Model file for the job. Use its own axes, mm. A direction names the side the tool comes from. Round coordinates to 2 decimals unless told otherwise and drop trailing zeros. Loops run counter-clockwise (first coordinate to the right, second up) from the corner with the lowest first, then second, coordinate; pieces in that order, holes last. Notation, with made-up numbers: (6.25, -11.75) - (37.25, -11.75) arc R20 cw to (37.25, 15.25) - close; hole circle Ø8 at (68, 87.25). An arc over 180 degrees is marked (long way). Answer as a JSON object with one key per item and string values.
from build123d import *

# Parameters (mm, degrees)
F0_R     = 3
F0_R_2   = 1.9
F0_R_3   = 1.2
F1_DEPTH = 2
F2_R     = 3
F2_R_2   = 1.9
F3_DEPTH = 1
F4_R     = 3
F5_DEPTH = 0.5
F6_R     = 3
F7_DEPTH = 3
F8_DEPTH = 5


with BuildPart() as f1:
    # F0 (on Top) → F1 (new body)
    with BuildSketch(Plane.XY):
        with Locations((-10.4432452041, 0)):
            Circle(F0_R)
        with Locations((-10.4432452041, 0)):
            Circle(F0_R_2, mode=Mode.SUBTRACT)
        with Locations((-10.4432452041, 0)):
            Circle(F0_R_2)
        with Locations((-10.4432452041, 0)):
            Circle(F0_R_3, mode=Mode.SUBTRACT)
        with Locations((-10.4432452041, 0)):
            Circle(F0_R_3)
    extrude(amount=F1_DEPTH)

    # F2 (on face) → F3 (join)
    with BuildSketch(Plane.XY.offset(2)):
        with Locations((-10.4432452041, 0)):
            Circle(F2_R)
        with Locations((-10.4432452041, 0)):
            Circle(F2_R_2, mode=Mode.SUBTRACT)
    extrude(amount=F3_DEPTH)

    # F4 (on face) → F5 (join)
    with BuildSketch(Plane.XY.offset(3)):
        with Locations((-10.4432452041, 0)):
            Circle(F4_R)
        with BuildLine():
            ThreePointArc((-12.2866257343, 0.4603783455), (-10.4432452041, 1.9), (-8.5998646739, 0.4603783455))
            Line((-8.5998646739, 0.4603783455), (-7.8815174605, 0.4603783455))
            Line((-7.8815174605, 0.4603783455), (-7.8815174605, -0.4603783455))
            Line((-7.8815174605, -0.4603783455), (-8.5998646739, -0.4603783455))
            ThreePointArc((-8.5998646739, -0.4603783455), (-10.4432452041, -1.9), (-12.2866257343, -0.4603783455))
            Line((-12.2866257343, -0.4603783455), (-12.7640617396, -0.4603783455))
            Line((-12.7640617396, -0.4603783455), (-12.7640617396, 0.4603783455))
            Line((-12.7640617396, 0.4603783455), (-12.2866257343, 0.4603783455))
        make_face(mode=Mode.SUBTRACT)
        with BuildLine():
            ThreePointArc((-12.2866257343, -0.4603783455), (-12.3432452041, 0), (-12.2866257343, 0.4603783455))
            Line((-12.2866257343, 0.4603783455), (-12.7640617396, 0.4603783455))
            Line((-12.7640617396, 0.4603783455), (-12.7640617396, -0.4603783455))
            Line((-12.7640617396, -0.4603783455), (-12.2866257343, -0.4603783455))
        make_face()
        with BuildLine():
            ThreePointArc((-11.5514201808, -0.4603783455), (-11.6432452041, 0), (-11.5514201808, 0.4603783455))
            Line((-11.5514201808, 0.4603783455), (-12.2866257343, 0.4603783455))
            ThreePointArc((-12.2866257343, 0.4603783455), (-12.3432452041, 0), (-12.2866257343, -0.4603783455))
            Line((-12.2866257343, -0.4603783455), (-11.5514201808, -0.4603783455))
        make_face()
        with BuildLine():
            ThreePointArc((-9.3350702274, -0.4603783455), (-9.2664253428, -0.234723271), (-9.2432452041, 0))
            ThreePointArc((-9.2432452041, 0), (-9.2664253428, 0.234723271), (-9.3350702274, 0.4603783455))
            Line((-9.3350702274, 0.4603783455), (-11.5514201808, 0.4603783455))
            ThreePointArc((-11.5514201808, 0.4603783455), (-11.6432452041, 0), (-11.5514201808, -0.4603783455))
            Line((-11.5514201808, -0.4603783455), (-9.3350702274, -0.4603783455))
        make_face()
        with BuildLine():
            Line((-11.5514201808, 0.4603783455), (-9.3350702274, 0.4603783455))
            ThreePointArc((-9.3350702274, 0.4603783455), (-10.4432452041, 1.2), (-11.5514201808, 0.4603783455))
        make_face()
        with BuildLine():
            ThreePointArc((-11.5514201808, -0.4603783455), (-10.4432452041, -1.2), (-9.3350702274, -0.4603783455))
            Line((-9.3350702274, -0.4603783455), (-11.5514201808, -0.4603783455))
        make_face()
        with BuildLine():
            ThreePointArc((-9.3350702274, 0.4603783455), (-9.2664253428, 0.234723271), (-9.2432452041, 0))
            ThreePointArc((-9.2432452041, 0), (-9.2664253428, -0.234723271), (-9.3350702274, -0.4603783455))
            Line((-9.3350702274, -0.4603783455), (-8.5998646739, -0.4603783455))
            ThreePointArc((-8.5998646739, -0.4603783455), (-8.5574531944, -0.2319234708), (-8.5432452041, 0))
            ThreePointArc((-8.5432452041, 0), (-8.5574531944, 0.2319234708), (-8.5998646739, 0.4603783455))
            Line((-8.5998646739, 0.4603783455), (-9.3350702274, 0.4603783455))
        make_face()
        with BuildLine():
            Line((-7.8815174605, 0.4603783455), (-8.5998646739, 0.4603783455))
            ThreePointArc((-8.5998646739, 0.4603783455), (-8.5574531944, 0.2319234708), (-8.5432452041, 0))
            ThreePointArc((-8.5432452041, 0), (-8.5574531944, -0.2319234708), (-8.5998646739, -0.4603783455))
            Line((-8.5998646739, -0.4603783455), (-7.8815174605, -0.4603783455))
            Line((-7.8815174605, -0.4603783455), (-7.8815174605, 0.4603783455))
        make_face()
    extrude(amount=F5_DEPTH)

    # F6 (on face) → F7 (join)
    with BuildSketch(Plane.XY.offset(3.5)):
        with Locations((-10.4432452041, 0)):
            Circle(F6_R)
        with BuildLine():
            ThreePointArc((-12.2866257343, 0.4603783455), (-10.4432452041, 1.9), (-8.5998646739, 0.4603783455))
            ThreePointArc((-8.5998646739, 0.4603783455), (-8.5574531944, 0.2319234708), (-8.5432452041, 0))
            ThreePointArc((-8.5432452041, 0), (-8.5574531944, -0.2319234708), (-8.5998646739, -0.4603783455))
            ThreePointArc((-8.5998646739, -0.4603783455), (-10.4432452041, -1.9), (-12.2866257343, -0.4603783455))
            ThreePointArc((-12.2866257343, -0.4603783455), (-12.3432452041, 0), (-12.2866257343, 0.4603783455))
        make_face(mode=Mode.SUBTRACT)
        with BuildLine():
            ThreePointArc((-9.3350702274, -0.4603783455), (-9.2664253428, -0.234723271), (-9.2432452041, 0))
            ThreePointArc((-9.2432452041, 0), (-9.2664253428, 0.234723271), (-9.3350702274, 0.4603783455))
            ThreePointArc((-9.3350702274, 0.4603783455), (-10.4432452041, 1.2), (-11.5514201808, 0.4603783455))
            ThreePointArc((-11.5514201808, 0.4603783455), (-11.6432452041, 0), (-11.5514201808, -0.4603783455))
            ThreePointArc((-11.5514201808, -0.4603783455), (-10.4432452041, -1.2), (-9.3350702274, -0.4603783455))
        make_face()
    extrude(amount=F7_DEPTH)

    # F8 (add): a face of the model
    f8_faces = [f1.faces().sort_by_distance(p)[0] for p in [
        (-10.4432452041, 0, 6.5),
    ]]
    extrude(f8_faces, amount=F8_DEPTH)


solid = f1.part
1) Slice it at D-D on z = 11.25. List the corners of the cut face in (x, y).
Values follow:
{"outline": "circle Ø2.4 at (-10.44, 0)"}
2) Two-plate mould, pull along X, no slides. Class faces 1 (the flat face through (-8, 0, 6.5)), 2 (the cylindrical face through (-11.643, -0.001, 7.19)), 3 (the cylindrical face through (-11.09, -2.93, 3.2)), 4 (the flat face through (-10, 0, 3)): pulls with the +X half, pulls with the -X half, needs draft (parallel to the pull), parting line crosses it, or undercut.
Values follow:
{"face 1": "needs draft", "face 2": "undercut", "face 3": "parting line crosses it", "face 4": "undercut"}
3) Slice it at C-C on x = -9.65. List the corners of the cut face in (y, z), then the cut area to 3 significant figures.
Values follow:
{"outline": "(-2.89, 0) - (2.89, 0) - (2.89, 6.5) - (1.73, 6.5) - (1.73, 2) - (-1.73, 2) - (-1.73, 6.5) - (-2.89, 6.5) - close; (-0.9, 3) - (0.9, 3) - (0.9, 11.5) - (-0.9, 11.5) - close", "area": "37.4 mm²"}
4) Probe probe 1 along Z at (x, y) = (-12.1, 0.4); probe 2 along Y at (x, z) = (-9.7, 4); probe 3 along Z at (x, y) = (-12.35, 1.1). List the from-to ranges inside material, lowest first.
Values follow:
{"probe 1": "0 to 2, 3 to 3.5", "probe 2": "-2.91 to -1.75, -0.94 to 0.94, 1.75 to 2.91", "probe 3": "0 to 6.5"}
5) Tool access for faces 5 (the flat face through (-10, 0, 2)), 6 (the flat face through (-10, 0, 11.5)): list every direction of +Z, -Z, +X, -X, +Y, -Y with a clear straight run to the whole face (end or side of a thin tool).
Values follow:
{"face 5": "none", "face 6": "+Z, +X, -X, +Y, -Y"}
6) Slice it at A-A on z = 6. List the corners of the cut face in (x, y).
Values follow:
{"outline": "circle Ø6 at (-10.44, 0); circle Ø2.4 at (-10.44, 0); hole circle Ø3.8 at (-10.44, 0)"}
7) Drop flat-ended pins along their axis: P1, Ø1, axis at y = -0.5, z = 10.5, coming from the -X side; P2, Ø0.7, axis at x = -11, y = -0.5, coming from the -Z side. Give the stop position or say it passes through.
Values follow:
{"P1": "x = -11.64", "P2": "z = 0"}
8) Slice it at B-B on y = -0.8. List the corners of the cut face in (x, z), then the cut area to 3 significant figures.
Values follow:
{"outline": "(-13.33, 0) - (-7.55, 0) - (-7.55, 6.5) - (-8.72, 6.5) - (-8.72, 2) - (-12.17, 2) - (-12.17, 6.5) - (-13.33, 6.5) - close; (-11.34, 3) - (-9.55, 3) - (-9.55, 11.5) - (-11.34, 11.5) - close", "area": "37.3 mm²"}
